Geometry check sheet. Reference: drawing and pictorial views, mm from the part's lowest x, y, z. A direction names the side the tool comes from. Give positions to 0.01 mm unless a question says otherwise; leave off trailing zeros. Order: outer loops, then holes, each group sorted by start corner. A loop starts at its lowest first (then second) coordinate and runs counter-clockwise, first axis right, second up. Notation, with made-up numbers: M 72.5,-37 L 78.5,-37 A22 cw 78.5,-5 Z; hole C 64.25,-10 d1. An arc over 180 degrees is marked long. Use CSV: the item, a comma, the result in double quotes. Start each with the question number.
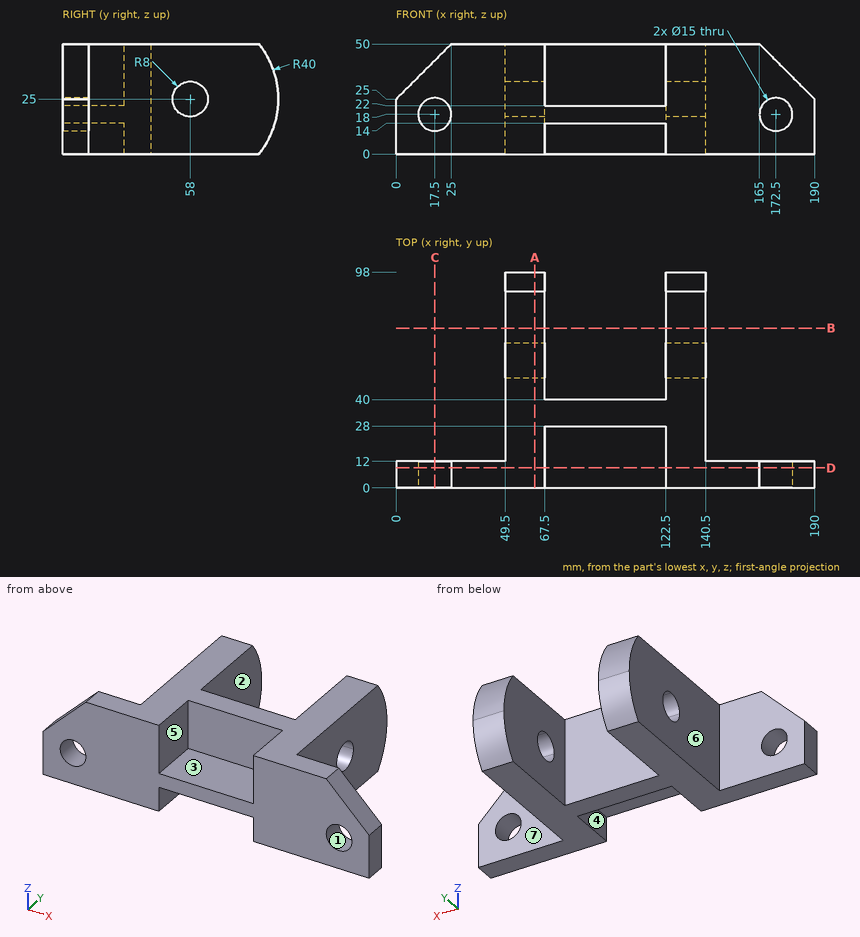
(1) Sectioned sample at B-B on y = 72.5. Record the cut outline in (x, z), then the cut area to 3 significant figures.
(2) Access from +Z, -Z, +X, -X, +Y, -Y to the whole of each face (thin tool, end or side, straight path). Record for the marked faces 4, 5, 6 and 7.
(3) Draft check along Z on the marked faces 1, 2 and 3. Enter one of: +Z half, -Z half, draft (parallel to the pull), parting line (faces both ways), or undercut.
(4) Sectioned sample at A-A on x = 63. Record the cut outline in (y, z), then the cut area to 3 significant figures.
(5) Sectioned sample at C-C on x = 17.5. Record the cut outline in (y, z).
(6) Thickness scan on line 1 (X direction, y = 9, z = 18); line 2 (X direction, y = 68, z = 14); line 3 (Y direction, x = 150.5, z = 18.5). Record the ranges inside material, lowest first.
(7) Sectioned sample at D-D on y = 9. Record the cut outline in (x, z), then the cut area to 3 significant figures.
(8) Go/stop test with flat-tipped pins: P1, Ø25, axis at x = 89.5, z = 28.5, coming from the +Y side; P2, Ø10, axis at y = 43, z = 36.5, coming from the -X side; P3, Ø4, axis at y = 16.5, z = 9, coming from the +X side; P4, Ø9, axis at x = 172.5, z = 18, coming from the -Y side. Record where each tip stops, or that it passes through.
Responses:
1,outline,"M 49.5,0 L 67.5,0 L 67.5,50 L 49.5,50 Z; M 122.5,0 L 140.5,0 L 140.5,50 L 122.5,50 Z"
1,area,"1,800 mm2"
2,face 4,"-Z, -Y"
2,face 5,"+Z, -Y"
2,face 6,"+Z, -Z, -X, +Y"
2,face 7,"+Z, -Z, +X, +Y"
3,face 1,"undercut"
3,face 2,"draft"
3,face 3,"+Z half"
4,outline,"M 0,0 L 89.22,0 A40 ccw 89.22,50 L 0,50 Z; hole C 58,25 d16"
4,area,"4,560 mm2"
5,outline,"M 0,0 L 12,0 L 12,10.5 L 0,10.5 Z; M 0,25.5 L 12,25.5 L 12,42.5 L 0,42.5 Z"
6,line 1,"0 to 10, 25 to 165, 180 to 190"
6,line 2,"49.5 to 67.5, 122.5 to 140.5"
6,line 3,"0 to 12"
7,outline,"M 0,0 L 67.5,0 L 67.5,14 L 122.5,14 L 122.5,0 L 190,0 L 190,25 L 165,50 L 122.5,50 L 122.5,22 L 67.5,22 L 67.5,50 L 25,50 L 0,25 Z; hole C 17.5,18 d15; hole C 172.5,18 d15"
7,area,"6,210 mm2"
8,P1,"y = 40"
8,P2,"x = 49.5"
8,P3,"x = 140.5"
8,P4,"through"
